from build123d import *

# Parameters (mm, degrees)
SKETCH1_W            = 139.7
SKETCH1_H            = 12.7
BOSS_EXTRUDE1_DEPTH  = 6.35
M3_CLEARANCE_HOLE1_D = 3.4
LPATTERN1_COUNT      = 4
LPATTERN1_PITCH      = 15.24
LPATTERN2_COUNT      = 4
LPATTERN2_PITCH      = 15.24


with BuildPart() as part:
    # Sketch1 → Boss-Extrude1 (new body)
    with BuildSketch(Plane.XY):
        Rectangle(SKETCH1_W, SKETCH1_H)
    extrude(amount=BOSS_EXTRUDE1_DEPTH)

    # M3 Clearance Hole1 (through all)
    with Locations(Plane(origin=(0, -6.35, 0), x_dir=(-1, 0, 0), z_dir=(0, -1, 0))):
        with Locations((65.0875, -3.175)):
            m3_clearance_hole1 = Hole(M3_CLEARANCE_HOLE1_D / 2)

    # Mirror1: M3 Clearance Hole1 across plane
    add(m3_clearance_hole1.mirror(Plane(origin=(0, 0, 0), x_dir=(0, 0, 1), z_dir=(1, 0, 0))), mode=Mode.SUBTRACT)

    # Sketch9 → Cut-Revolve1 (revolve, cut)
    with BuildSketch(Plane(origin=(0, 6.35, 0), x_dir=(1, 0, 0), z_dir=(0, 1, 0))):
        Polygon((2.5, -5.55625), (2.921, -5.55625), (2.921, -4.34975), (2.5, -4.34975), (2.5, 0), (0, 0), (0, -6.35), (2.5, -6.35), align=None)
    cut_revolve1 = revolve(axis=Axis((0, 6.35, 0), (0, 0, 1)), mode=Mode.SUBTRACT)

    # LPattern1: Cut-Revolve1 ×4
    with Locations(*[(-i * LPATTERN1_PITCH, 0, 0) for i in range(1, LPATTERN1_COUNT)]):
        add(cut_revolve1, mode=Mode.SUBTRACT)

    # LPattern2: Cut-Revolve1 ×4
    with Locations(*[(i * LPATTERN2_PITCH, 0, 0) for i in range(1, LPATTERN2_COUNT)]):
        add(cut_revolve1, mode=Mode.SUBTRACT)


solid = part.part
Work out the finished part from the listing and answer in its coordinate system (mm). A direction names the side the tool comes from. Give positions to 0.01 mm unless a question says otherwise; leave off trailing zeros. Order: outer loops, then holes, each group sorted by start corner. A loop starts at its lowest first (then second) coordinate and runs counter-clockwise, first axis right, second up. Notation, with made-up numbers: (65.25, 53) -> (105.25, 53) arc R13 cw to (105.25, 68) -> close; hole circle Ø8 at (-28, 31.25). An arc over 180 degrees is marked (long way). Answer as a JSON object with one key per item and string values. Group by question number.
1. Section A-A on x = -15.24 is taken. Determine the outline of the cut face in (y, z), plus the area to 3 significant figures.
2. Section B-B on y = -0.75 is taken. Count the separate pieces of the cut face and the enclosed holes in it, plus the area to 3 significant figures.
3. Consider line 1 along X through (y, z) = (3, 2.75); line 2 along X through (y, z) = (0.25, 2); line 3 along Y through (x, z) = (30.5, 1.25). Determine where each line is inside the solid, lowest interval first. Write a range as [from, to].
4. A tool of negligible diameter and unlimited length cuts with its end or side. For faces 1 (the flat face through (-15, 3.7, 4.35)), 2 (the cylindrical face through (15.19, 3.85, 5.95)), from which of +Z, -Z, +X, -X, +Y, -Y can it reach the whole face along a straight path? Write none if from no direction.
5. A flat-ended cylindrical pin translates along its axis: pin 1 Ø2.5 at (x, y) = (45.5, 5.5) entering from +Z. Find the tip coordinate at first contact, or state that the pin passes through.
6. The mould has two halves that part along X. Classify faces 3 (the flat face through (30.7, 3.7, 4.35)), 4 (the flat face through (8, 6.35, 3)): released by +X, released by -X, zero draft, split by the parting line, or undercut.
Result sheet:
{
 "1": {"outline": "(-6.35, 0) -> (3.85, 0) -> (3.85, 4.35) -> (3.43, 4.35) -> (3.43, 5.56) -> (3.85, 5.56) -> (3.85, 6.35) -> (-6.35, 6.35) -> close", "area": "64.3 mm^2"},
 "2": {"separate pieces": "1", "enclosed holes": "2", "area": "869 mm^2"},
 "3": {"line 1": "x = [-69.85, -66.73], [-63.44, 63.44], [66.73, 69.85]", "line 2": "x = [-69.85, -66.32], [-63.86, 63.86], [66.32, 69.85]", "line 3": "y = [-6.35, 3.85]"},
 "4": {"face 1": "+Y", "face 2": "+Z, -Z, +Y"},
 "5": {"pin 1": "passes through"},
 "6": {"face 3": "undercut", "face 4": "zero draft"}
}
